Geometry: final body of the model. Coordinates: model frame, mm. A direction names the side the tool comes from. Give positions to 0.01 mm unless a question says otherwise; leave off trailing zeros. Write each loop counter-clockwise with the first axis right and the second up, starting at its lowest first coordinate (ties: lowest second). Pieces come first, ordered by that corner, then holes. Notation, with made-up numbers: M -29.75,-28.5 L -9.75,-28.5 A23 ccw -9.75,-4.5 Z; hole C 23.5,33.5 d10. An arc over 180 degrees is marked long. One line per question, with ' | ' between items.
from build123d import *

# Parameters (mm, degrees)
SKETCH_W        = 200
SKETCH_H        = 125
PAD_DEPTH       = 10
SKETCH001_W     = 177
SKETCH001_H     = 102
PAD001_DEPTH    = 2
POCKET_DEPTH    = 120
SKETCH003_W     = 85
SKETCH003_H     = 10
POCKET001_DEPTH = 12.001
FILLET_R        = 2
CHAMFER_SIZE    = 1
CHAMFER001_SIZE = 1
CHAMFER002_SIZE = 1


with BuildPart() as part:
    # Sketch → Pad (new body)
    with BuildSketch(Plane.XY):
        Rectangle(SKETCH_W, SKETCH_H)
    extrude(amount=PAD_DEPTH)

    # Sketch001 (on Face6 of Pad) → Pad001 (join)
    with BuildSketch(Plane.XY.offset(10)):
        Rectangle(SKETCH001_W, SKETCH001_H)
    extrude(amount=PAD001_DEPTH)

    # Sketch002 (on Face2 of Pad001) → Pocket (cut)
    with BuildSketch(Plane(origin=(-100, 0, 0), x_dir=(0, -1, 0), z_dir=(-1, 0, 0))):
        Polygon((-60.5, 0), (-56.964466, 3.535534), (-53.428932, 0), (-56.964466, -3.535534), align=None)
    extrude(amount=-POCKET_DEPTH, mode=Mode.SUBTRACT)

    # Sketch003 (on Face4 of Pocket) → Pocket001 (cut, through all)
    with BuildSketch(Plane(origin=(0, 0, 0), x_dir=(1, 0, 0), z_dir=(0, 0, -1))):
        with Locations((-57.5, -57.5)):
            Rectangle(SKETCH003_W, SKETCH003_H)
    extrude(amount=-POCKET001_DEPTH, mode=Mode.SUBTRACT)

    # Fillet
    fillet_edges = [part.edges().sort_by_distance(p)[0] for p in [
        (100, 62.5, 5),
    ]]
    fillet(fillet_edges, radius=FILLET_R)

    # Chamfer
    chamfer_edges = [part.edges().sort_by_distance(p)[0] for p in [
        (100, -1, 0),
    ]]
    chamfer(chamfer_edges, length=CHAMFER_SIZE)

    # Chamfer001
    chamfer001_edges = [part.edges().sort_by_distance(p)[0] for p in [
        (-100, -5, 0),
    ]]
    chamfer(chamfer001_edges, length=CHAMFER001_SIZE)

    # Chamfer002
    chamfer002_edges = [part.edges().sort_by_distance(p)[0] for p in [
        (0, -62.5, 0),
    ]]
    chamfer(chamfer002_edges, length=CHAMFER002_SIZE)


solid = part.part
(1) Cut plane B-B, the plane x = 32. Return loops of the section in (y, z), then the cut area to 3 significant figures.
Working result:
outline: M -62.5,1 L -61.5,0 L 61.5,0 L 62.5,1 L 62.5,10 L 51,10 L 51,12 L -51,12 L -51,10 L -62.5,10 Z | area: 1,450 mm^2
(2) Cut plane C-C, the plane z = 8. Return loops of the section in (x, y), then the cut area to 3 significant figures.
Working result:
outline: M -100,-62.5 L 100,-62.5 L 100,60.5 A2 ccw 98,62.5 L -15,62.5 L -15,52.5 L -100,52.5 Z | area: 24,100 mm^2
(3) Material intervals for L1, parallel to Y at x = -82, z = 3.25; L2, parallel to Z at x = 29.5, y = 56.5; L3, parallel to X at y = 53, z = 8, sorted ascending. Write a range as [from, to].
Working result:
L1: y = [-62.5, 52.5] | L2: z = [0, 10] | L3: x = [-15, 100]
(4) First-contact query: P1, Ø1.6, axis at y = 3, z = 11, coming from the +X side; P2, Ø3, axis at y = 58.5, z = 1.5, coming from the -X side; P3, Ø1, axis at x = -6, z = 11, coming from the +Y side. Flat tips, straight axial feed; report the tip coordinate or a pass-through.
Working result:
P1: stops at x = 88.5 | P2: stops at x = -15 | P3: stops at y = 51
(5) Cut plane A-A, the plane y = -23. Return loops of the section in (x, z), then the cut area to 3 significant figures.
Working result:
outline: M -100,1 L -99,0 L 99,0 L 100,1 L 100,10 L 88.5,10 L 88.5,12 L -88.5,12 L -88.5,10 L -100,10 Z | area: 2,350 mm^2
(6) Set-up query: faces 1 (the face through (-15, 58, 6)), 2 (the face through (-1, 1, 0)). Return all of +Z, -Z, +X, -X, +Y, -Y with unobstructed straight access to the full face (end or side cutting, diameter ignored); none if empty.
Working result:
face 1: +Z, -Z, -X, +Y | face 2: -Z, +X, -X, +Y, -Y
(7) Cut plane D-D, the plane y = -54. Return loops of the section in (x, z).
Working result:
outline: M -100,1 L -99,0 L 99,0 L 100,1 L 100,10 L -100,10 Z
